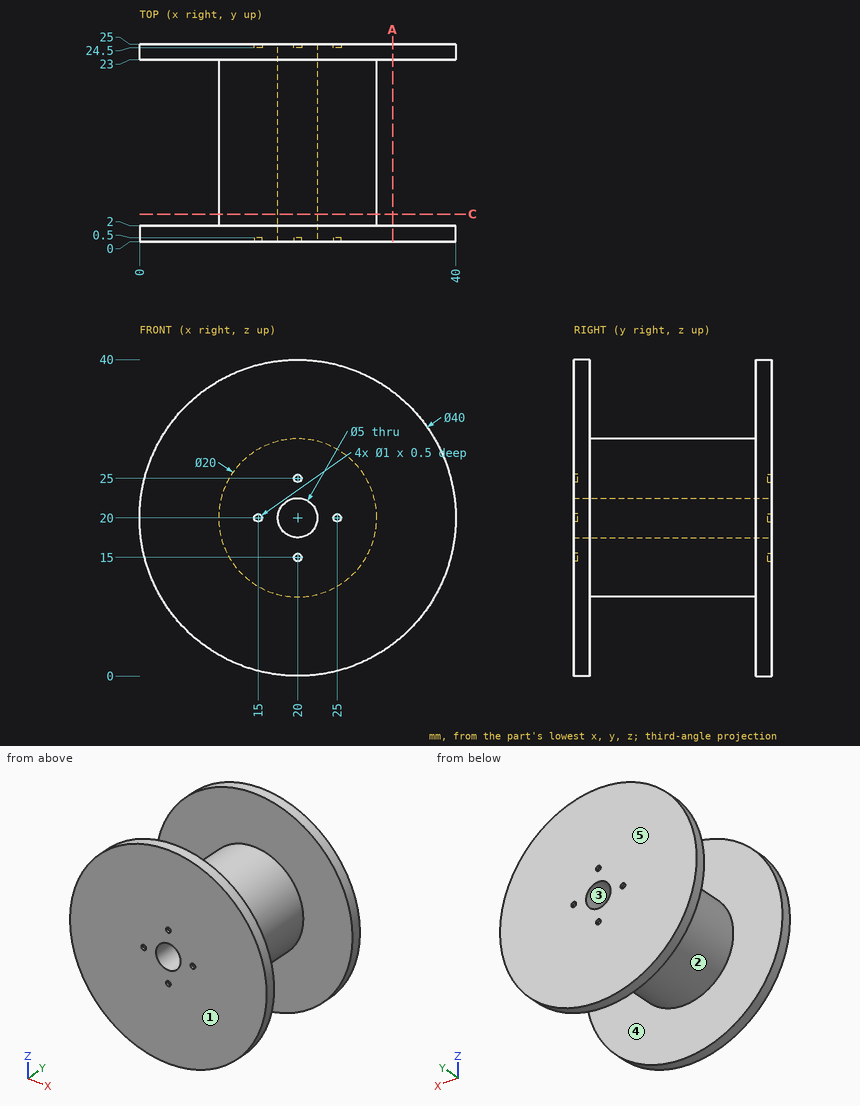
Can you work these out from the drawing? Everything is in mm from the part's minimum corner. A direction names the side the tool comes from. Coordinates: 2 decimals unless noted, no trailing zeros. Order: outer loops, then holes, each group sorted by start corner. A loop starts at its lowest first (then second) coordinate and runs counter-clockwise, first axis right, second up. Notation, with made-up numbers: M -14,-22 L 18,-22 A10 ccw 18,-10 Z; hole C 68,76 d8. An arc over 180 degrees is marked long. Answer as CSV lines item,"result". Start each with the question number.
1. I want a section at A-A, the plane x = 32. Write out the boundary of the cut face in (y, z), and give its area (3 significant figures).
2. I need wall thicknesses on line 1 (X direction, y = 24.9, z = 20); line 2 (Y direction, x = 34, z = 14); line 3 (Z direction, x = 20, y = 17.25). Which ranges of each line are inside material? Lowest first, please. Write a range as [from, to].
3. For pin 1 (12 mm diameter, centred on y = 11.5, z = 30.5, fed in from +X); pin 2 (0.8 mm diameter, centred on x = 20, z = 15, fed in from +Y); pin 3 (6 mm diameter, centred on x = 9.5, y = 20.5, fed in from -Z); pin 4 (4.5 mm diameter, centred on x = 20, z = 20, fed in from -Y), each with a flat end and sliding along its axis, tell me the tip position at first contact or that it passes through.
4. We'd pull the mould along Y, two halves only. Please class the marked faces 1, 2 and 3: released by +Y, released by -Y, zero draft, split by the parting line, or undercut.
5. On a 3-axis mill with a long thin cutter (end or side, diameter ignored), from which of +Z, -Z, +X, -X, +Y, -Y can I reach the whole of each face in a straight line? I mean the marked faces 4 and 5. Say none if no direction works.
6. I want a section at C-C, the plane y = 3.5. Write out the boundary of the cut face in (x, z).
Recorded:
1,outline,"M 0,4 L 2,4 L 2,36 L 0,36 Z; M 23,4 L 25,4 L 25,36 L 23,36 Z"
1,area,"128 mm2"
2,line 1,"x = [0, 14.5], [15.5, 17.5], [22.5, 24.5], [25.5, 40]"
2,line 2,"y = [0, 2], [23, 25]"
2,line 3,"z = [10, 17.5], [22.5, 30]"
3,pin 1,"stops at x = 28.93"
3,pin 2,"stops at y = 24.5"
3,pin 3,"stops at z = 2.06"
3,pin 4,"passes through"
4,face 1,"released by -Y"
4,face 2,"undercut"
4,face 3,"zero draft"
5,face 4,"none"
5,face 5,"+Z, -Z, +X, -X, +Y"
6,outline,"C 20,20 d20; hole C 20,20 d5"
